Model file for the job. Use its own axes, mm. A direction names the side the tool comes from. Coordinates: 2 decimals unless noted, no trailing zeros. Write each loop counter-clockwise with the first axis right and the second up, starting at its lowest first coordinate (ties: lowest second). Pieces come first, ordered by that corner, then holes. Notation, with made-up numbers: (-33, -4.5) - (3, -4.5) arc R17 ccw to (3, 6.5) - close; hole circle Ø1 at (4.5, 12). An arc over 180 degrees is marked (long way). Put each result on its own line as item: value. Start each with the question number.
1. Saw through at B-B, the plane x = -6. Write the cut outline in (y, z).
2. Saw through at D-D, the plane x = -1.5. Write the cut outline in (y, z).
3. Saw through at C-C, the plane z = 3. Write the cut outline in (x, y), plus the area to 3 significant figures.
4. Drill centre lines: L1, parallel to Z at x = -6, y = -2.5; L2, parallel to Y at x = 0.5, z = 32; L3, parallel to Z at x = -3.5, y = 4.75. Where is each one in solid material? Low to high. Write a range as from..to.
5. Pull direction Z, two halves, no side cores. Call faces 1 (the face through (0.54, -2.44, -2.46)), 2 (the face through (2, -2, 0)), 3 (the face through (0, 0, 10)), 4 (the face through (2.76, 4.27, 27.12)): released by +Z, released by -Z, zero draft, split by the parting line, or undercut.
6. Drop flat-ended pins along their axis: P1, Ø1, axis at y = 4, z = 19, coming from the +X side; P2, Ø4, axis at x = -3.67, z = 26.97, coming from the -Y side; P3, Ø1, axis at x = 5, z = 3.5, coming from the -Y side. Give the stop position or say it passes through.
7. Saw through at A-A, the plane y = 0. Write the cut outline in (x, z).
8. Which spindle directions (+Z, -Z, +X, -X, +Y, -Y) get a long thin tool onto all of the face, cutting with end or side? Do faces 5 (the face through (0, 6, 22)), 6 (the face through (0, 2.5, 22)), 7 (the face through (7.14, 4, 20)). Say none if no direction does.
```python
from build123d import *

# Parameters (mm, degrees)
CROQUIS1_R              = 15
SALIENTE_EXTRUIR1_DEPTH = 10
CROQUIS2_R              = 2.5
SALIENTE_EXTRUIR3_DEPTH = 5
CROQUIS3_W              = 27.214568237
CROQUIS3_H              = 3.5
SALIENTE_EXTRUIR5_DEPTH = 30
REDONDEO1_SIZE          = 10
REDONDEO2_SIZE          = 10
CROQUIS4_R              = 1.2
CORTAR_EXTRUIR7_DEPTH   = 30
CORTAR_EXTRUIR8_DEPTH   = 30
CORTAR_EXTRUIR9_START   = -30
CROQUIS8_R              = 15
CROQUIS8_R_2            = 10
CORTAR_EXTRUIR9_DEPTH   = 30
CROQUIS9_R              = 1.239789427
CROQUIS9_R_2            = 1.228877731
SALIENTE_EXTRUIR6_DEPTH = 3.5
CROQUIS10_R             = 1.2
CORTAR_EXTRUIR11_DEPTH  = 3.5


with BuildPart() as part:
    # Croquis1 → Saliente-Extruir1 (new body)
    with BuildSketch(Plane.XY):
        Circle(CROQUIS1_R)
    extrude(amount=SALIENTE_EXTRUIR1_DEPTH)

    # Croquis2 → Saliente-Extruir3 (add)
    with BuildSketch(Plane(origin=(0, 0, 0), x_dir=(-1, 0, 0), z_dir=(0, 0, -1))):
        Circle(CROQUIS2_R)
    extrude(amount=SALIENTE_EXTRUIR3_DEPTH)

    # Croquis3 → Saliente-Extruir5 (add)
    with BuildSketch(Plane.XY.offset(10)):
        with Locations((0.140442967, 4.25)):
            Rectangle(CROQUIS3_W, CROQUIS3_H)
    extrude(amount=SALIENTE_EXTRUIR5_DEPTH)

    # Redondeo1
    redondeo1_edges = [part.edges().sort_by_distance(p)[0] for p in [
        (13.747727085, 4.25, 40),
    ]]
    chamfer(redondeo1_edges, length=REDONDEO1_SIZE)

    # Redondeo2
    redondeo2_edges = [part.edges().sort_by_distance(p)[0] for p in [
        (-13.466841152, 4.25, 40),
    ]]
    chamfer(redondeo2_edges, length=REDONDEO2_SIZE)

    # Croquis4 → Cortar-Extruir7 (cut)
    with BuildSketch(Plane(origin=(0, 6, 0), x_dir=(1, 0, 0), z_dir=(0, 1, 0))):
        with Locations(Location((-2.669557034, -26.064684959, 0), (0, 0, 270))):
            Circle(CROQUIS4_R)
        with Locations(Location((2.950442966, -26.064684959, 0), (0, 0, 270))):
            Circle(CROQUIS4_R)
    extrude(amount=-CORTAR_EXTRUIR7_DEPTH, mode=Mode.SUBTRACT)

    # Croquis7 → Cortar-Extruir8 (cut)
    with BuildSketch(Plane(origin=(0, 6, 0), x_dir=(1, 0, 0), z_dir=(0, 1, 0))):
        Polygon((-6.859557034, -30.106136843), (-6.859557034, -22.023233074), (-6.859557034, -10), (-13.466841152, -10), (-13.466841152, -30), (-3.466841152, -40), (3.747727085, -40), (13.747727085, -30), (13.747727085, -10), (7.140442966, -10), (7.140442966, -22.023233074), (7.140442966, -30.106136843), (0.140442966, -34.147588727), align=None)
    extrude(amount=-CORTAR_EXTRUIR8_DEPTH, mode=Mode.SUBTRACT)

    # Croquis8 → Cortar-Extruir9 (cut)
    with BuildSketch(Plane.XY.offset(10).offset(CORTAR_EXTRUIR9_START)):
        Circle(CROQUIS8_R)
        Circle(CROQUIS8_R_2, mode=Mode.SUBTRACT)
    extrude(amount=CORTAR_EXTRUIR9_DEPTH, mode=Mode.SUBTRACT)

    # Croquis9 → Saliente-Extruir6 (add)
    with BuildSketch(Plane(origin=(0, 6, 0), x_dir=(1, 0, 0), z_dir=(0, 1, 0))):
        with Locations((-2.669557034, -26.064684959)):
            Circle(CROQUIS9_R)
        with Locations((2.950442966, -26.064684959)):
            Circle(CROQUIS9_R_2)
    extrude(amount=-SALIENTE_EXTRUIR6_DEPTH)

    # Croquis10 → Cortar-Extruir11 (cut)
    with BuildSketch(Plane(origin=(0, 6, 0), x_dir=(1, 0, 0), z_dir=(0, 1, 0))):
        with Locations(Location((-3.669557034, -26.965113623, 0), (0, 0, 270))):
            Circle(CROQUIS10_R)
        with Locations(Location((3.950442966, -26.965113623, 0), (0, 0, 90))):
            Circle(CROQUIS10_R)
    extrude(amount=-CORTAR_EXTRUIR11_DEPTH, mode=Mode.SUBTRACT)


solid = part.part
```
Final values:
1. outline: (-8, 0) - (8, 0) - (8, 10) - (6, 10) - (6, 30.6) - (2.5, 30.6) - (2.5, 10) - (-8, 10) - close
2. outline: (-9.89, 0) - (-2, 0) - (-2, -5) - (2, -5) - (2, 0) - (9.89, 0) - (9.89, 10) - (6, 10) - (6, 33.2) - (2.5, 33.2) - (2.5, 10) - (-9.89, 10) - close
3. outline: circle Ø20 at (0, 0)
3. area: 314 mm²
4. L1: z = 0..10
4. L2: y = 2.5..6
4. L3: z = 0..25.78, 28.15..32.05
5. face 1: zero draft
5. face 2: released by -Z
5. face 3: released by +Z
5. face 4: undercut
6. P1: stops at x = 7.14
6. P2: stops at y = 2.5
6. P3: stops at y = -8.93
7. outline: (-10, 0) - (-2.5, 0) - (-2.5, -5) - (2.5, -5) - (2.5, 0) - (10, 0) - (10, 10) - (-10, 10) - close
8. face 5: +Z, +X, -X, +Y
8. face 6: +Z, +X, -X, -Y
8. face 7: +Z, +X, +Y, -Y
